Geometry: see drawing. Coordinates: mm, zero at the bounding-box minimum. Give positions to 0.01 mm unless a question says otherwise; leave off trailing zeros. Write each loop counter-clockwise with the first axis right and the second up, starting at its lowest first coordinate (ties: lowest second). Pieces come first, ordered by that corner, then holes. Notation, with made-up numbers: M 8.5,74.5 L 44.5,74.5 A24 cw 44.5,101.5 Z; hole C 65,45 d6. An arc over 180 degrees is marked long. Use a Markdown table: item, result. Add a question column.
(1) Draft query along Y for the marked faces 1, 2 and 3. Return one class per face: released by +Y, released by -Y, zero draft, split by the parting line, or undercut.
(2) Cut plane D-D (y = 22). Output: boundary loops of the cut face in (x, z).
(3) Pin query (flat end, axial travel): pin 1 Ø8.5 at (x, y) = (170, 19.7) entering from -Z. Return the tip coordinate at first contact, or that it passes through.
(4) Cut plane C-C (x = 170). Output: boundary loops of the cut face in (y, z), plus the area to 3 significant figures.
(5) Cut plane B-B (z = 7). Output: boundary loops of the cut face in (x, y), plus the area to 3 significant figures.
(6) Cut plane A-A (x = 100). Output: boundary loops of the cut face in (y, z).
(7) Material intervals for L1, parallel to Y at x = 170, z = 9.25; L2, parallel to Y at x = 25, z = 8 (1 decimal); L3, parallel to X at y = 57, z = 9.75 (1 decimal), sorted ascending.
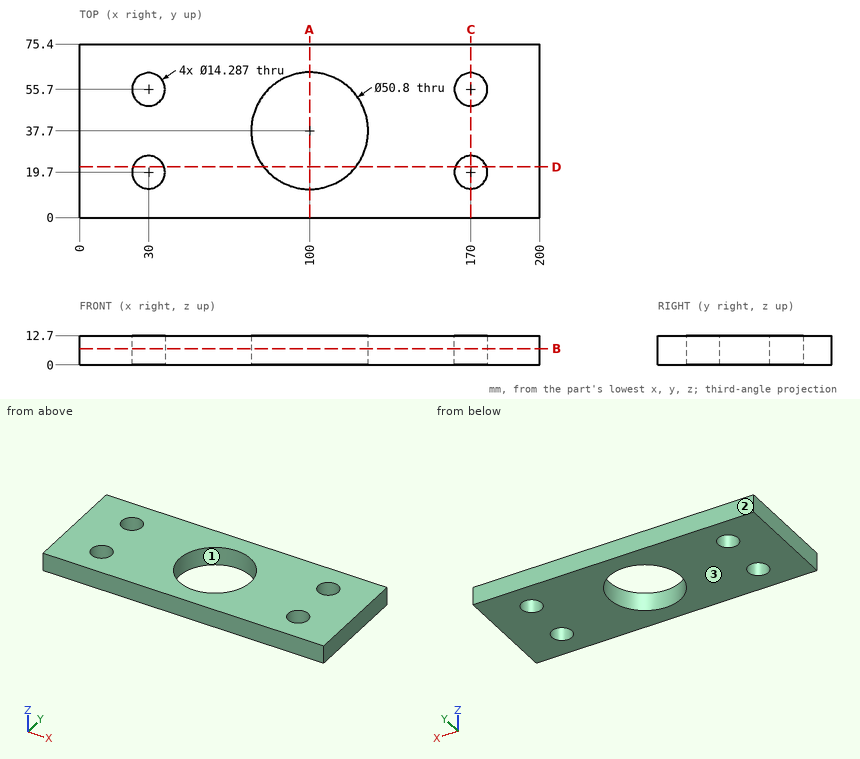
Answer list:
| question | item | result |
|---|---|---|
| 1 | face 1 | undercut |
| 1 | face 2 | released by +Y |
| 1 | face 3 | zero draft |
| 2 | outline | M 0,0 L 23.24,0 L 23.24,12.7 L 0,12.7 Z; M 36.76,0 L 80.03,0 L 80.03,12.7 L 36.76,12.7 Z; M 119.97,0 L 163.24,0 L 163.24,12.7 L 119.97,12.7 Z; M 176.76,0 L 200,0 L 200,12.7 L 176.76,12.7 Z |
| 3 | pin 1 | through |
| 4 | outline | M 0,0 L 12.56,0 L 12.56,12.7 L 0,12.7 Z; M 26.84,0 L 48.56,0 L 48.56,12.7 L 26.84,12.7 Z; M 62.84,0 L 75.4,0 L 75.4,12.7 L 62.84,12.7 Z |
| 4 | area | 595 mm² |
| 5 | outline | M 0,0 L 200,0 L 200,75.4 L 0,75.4 Z; hole C 30,19.7 d14.29; hole C 30,55.7 d14.29; hole C 100,37.7 d50.8; hole C 170,19.7 d14.29; hole C 170,55.7 d14.29 |
| 5 | area | 12,400 mm² |
| 6 | outline | M 0,0 L 12.3,0 L 12.3,12.7 L 0,12.7 Z; M 63.1,0 L 75.4,0 L 75.4,12.7 L 63.1,12.7 Z |
| 7 | L1 | 0 to 12.56, 26.84 to 48.56, 62.84 to 75.4 |
| 7 | L2 | 0 to 14.6, 24.8 to 50.6, 60.8 to 75.4 |
| 7 | L3 | 0 to 23, 37 to 83.5, 116.5 to 163, 177 to 200 |
